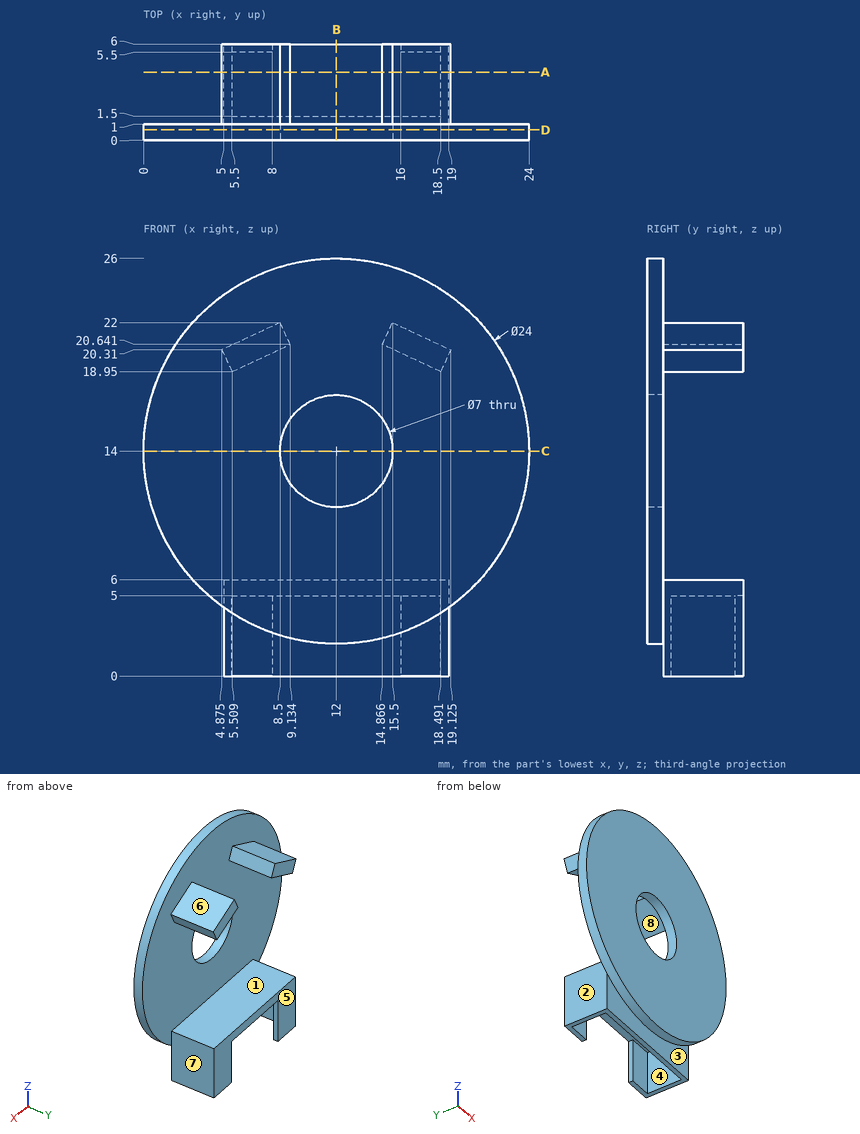
Part print with two shaded views. Sizes in mm from the minimum x, y, z corner. A direction names the side the tool comes from. Round coordinates to 2 decimals unless told otherwise and drop trailing zeros. Order: outer loops, then holes, each group sorted by start corner. A loop starts at its lowest first (then second) coordinate and runs counter-clockwise, first axis right, second up. Notation, with made-up numbers: (48.5, 26) - (89.5, 26) arc R15 ccw to (89.5, 49) - close; hole circle Ø9 at (3, 50). An arc over 180 degrees is marked (long way). Answer in a Markdown table with one row per item. Add a question column.
(1) Drop flat-ended pins along their axis: pin 1 Ø3 at (y, z) = (3, 1.5) entering from +X; pin 2 Ø9 at (x, z) = (12, 14) entering from +Y; pin 3 Ø2 at (x, y) = (9.5, 4.5) entering from -Z. Give the stop position or say it passes through.
(2) Mould opens along Z. For the marked faces 6, 7 and 8 say: +Z half, -Z half, draft (parallel to the pull), parting line (faces both ways), or undercut.
(3) 3-axis set-ups, long thin cutter, end or side, ignore diameter. For the marked faces 1, 2, 3, 4 and 5: which of +Z, -Z, +X, -X, +Y, -Y reach the whole face in a straight line?
(4) Band-saw the part on B-B on x = 12. List the corners of the cut face in (y, z).
(5) Probe L1, parallel to X at y = 1.7, z = 1; L2, parallel to X at y = 0.4, z = 14; L3, parallel to Z at x = 12, y = 0.5. List the from-to ranges inside material, lowest first. Write a range as [from, to].
(6) Band-saw the part on D-D on y = 0.65. List the corners of the cut face in (x, z), and give its area (3 significant figures).
(7) Band-saw the part on C-C on z = 14. List the corners of the cut face in (x, y).
(8) Band-saw the part on A-A on y = 4.25. Count the separate pieces of the cut face and the enclosed holes in it.
Data:
| question | item | result |
|---|---|---|
| 1 | pin 1 | stops at x = 19 |
| 1 | pin 2 | stops at y = 1 |
| 1 | pin 3 | stops at z = 5 |
| 2 | face 6 | +Z half |
| 2 | face 7 | draft |
| 2 | face 8 | undercut |
| 3 | face 1 | +X, -X, +Y |
| 3 | face 2 | -Z, -X, +Y |
| 3 | face 3 | -Z, -Y |
| 3 | face 4 | -Z |
| 3 | face 5 | +Z, -Z, +X, -X, +Y |
| 4 | outline | (0, 2) - (1, 2) - (1, 0) - (1.5, 0) - (1.5, 5) - (6, 5) - (6, 6) - (1, 6) - (1, 10.5) - (0, 10.5) - close; (0, 17.5) - (1, 17.5) - (1, 26) - (0, 26) - close |
| 5 | L1 | x = [5, 5.5], [18.5, 19] |
| 5 | L2 | x = [0, 8.5], [15.5, 24] |
| 5 | L3 | z = [2, 10.5], [17.5, 26] |
| 6 | outline | circle Ø24 at (12, 14); hole circle Ø7 at (12, 14) |
| 6 | area | 414 mm^2 |
| 7 | outline | (0, 0) - (8.5, 0) - (8.5, 1) - (0, 1) - close; (15.5, 0) - (24, 0) - (24, 1) - (15.5, 1) - close |
| 8 | separate pieces | 3 |
| 8 | enclosed holes | 0 |
